For this review, take the finished solid that the model builds, in its own axes (mm). A direction names the side the tool comes from. Round coordinates to 2 decimals unless told otherwise and drop trailing zeros. Loops run counter-clockwise (first coordinate to the right, second up) from the corner with the lowest first, then second, coordinate; pieces in that order, holes last.
1. Tool access review of faces 1 (the flat face through (-9, 4.5, 0)), 2 (the flat face through (-2, 26.7, 0)), 3 (the flat face through (15, 17, 0.65)): name each direction out of +Z, -Z, +X, -X, +Y, -Y from which nothing blocks a thin tool from reaching the whole face with its end or side.
2. Clearance check with flat-ended pins moving along their axes: pin 1 Ø2 at (y, z) = (23.5, 3) entering from -X; pin 2 Ø4.5 at (y, z) = (20, 2.5) entering from -X; pin 3 Ø6 at (x, z) = (4.5, 1) entering from +Y; pin 4 Ø1.4 at (x, z) = (-14.5, -2) entering from +Y. State where each tip first meets the part, or that it passes through.
3. To check wall thickness, follow line 1 along Y through (x, z) = (-10, 0.25); line 2 along Z through (x, y) = (-13.65, 17.2); line 3 along X through (y, z) = (17.15, 0). State the ranges of each line that lie inside material, in increasing order.
4. Consider section C-C on x = 0.95. State the section outline as (y, z) points, then the cut area to 3 significant figures.
5. Consider section D-D on y = 13.75. State the section outline as (x, z) points.
6. Consider section A-A on x = 13.65. State the section outline as (y, z) points, then the cut area to 3 significant figures.
7. Consider section B-B on z = -3.25. State the section outline as (x, y) points, then the cut area to 3 significant figures.
from build123d import *

# Parameters (mm, degrees)
SKETCH1_W           = 22.5
SKETCH1_H           = 11.8
BOSS_EXTRUDE1_DEPTH = 22.7
BOSS_EXTRUDE2_START = 15.9
SKETCH2_W           = 31.9
SKETCH2_H           = 11.8
BOSS_EXTRUDE2_DEPTH = 2.5
SKETCH3_R           = 1
CUT_EXTRUDE1_DEPTH  = 26.055388642
SKETCH4_R           = 5.9
SKETCH4_R_2         = 2.3
SKETCH4_R_3         = 2.5
BOSS_EXTRUDE3_DEPTH = 4
SKETCH4_3_R         = 2.3
BOSS_EXTRUDE4_DEPTH = 7.2
SKETCH5_W           = 3.6
SKETCH5_H           = 1.2
CUT_EXTRUDE2_DEPTH  = 4


with BuildPart() as part:
    # Sketch1 → Boss-Extrude1 (new body)
    with BuildSketch(Plane(origin=(0, 0, 0), x_dir=(1, 0, 0), z_dir=(0, 1, 0))):
        Rectangle(SKETCH1_W, SKETCH1_H)
    extrude(amount=BOSS_EXTRUDE1_DEPTH)

    # Sketch2 → Boss-Extrude2 (add)
    with BuildSketch(Plane(origin=(0, 0, 0), x_dir=(1, 0, 0), z_dir=(0, 1, 0)).offset(BOSS_EXTRUDE2_START)):
        Rectangle(SKETCH2_W, SKETCH2_H)
    extrude(amount=BOSS_EXTRUDE2_DEPTH)

    # Sketch3 → Cut-Extrude1 (cut, through all)
    with BuildSketch(Plane(origin=(0, 18.4, 0), x_dir=(1, 0, 0), z_dir=(0, 1, 0))):
        with BuildLine():
            Line((-14.409934208, 0.65), (-15.95, 0.65))
            Line((-15.95, 0.65), (-15.95, -0.65))
            Line((-15.95, -0.65), (-14.409934208, -0.65))
            ThreePointArc((-14.409934208, -0.65), (-14.65, 0), (-14.409934208, 0.65))
        make_face()
        with Locations((-13.65, 0)):
            Circle(SKETCH3_R)
        with Locations((13.65, 0)):
            Circle(SKETCH3_R)
        with BuildLine():
            Line((14.409934208, -0.65), (15.95, -0.65))
            Line((15.95, -0.65), (15.95, 0.65))
            Line((15.95, 0.65), (14.409934208, 0.65))
            ThreePointArc((14.409934208, 0.65), (14.588065618, 0.34645764), (14.65, 0))
            ThreePointArc((14.65, 0), (14.588065618, -0.34645764), (14.409934208, -0.65))
        make_face()
    extrude(amount=-CUT_EXTRUDE1_DEPTH, mode=Mode.SUBTRACT)

    # Sketch4 → Boss-Extrude3 (add)
    # profile 1 of 2: a face of its own
    with BuildSketch(Plane(origin=(0, 22.7, 0), x_dir=(1, 0, 0), z_dir=(0, 1, 0))):
        with Locations((-5.35, 0)):
            Circle(SKETCH4_R)
        with Locations(Location((-5.35, 0, 0), (0, 0, 270))):
            Circle(SKETCH4_R_2, mode=Mode.SUBTRACT)
    # profile 2 of 2: a face of its own
    with BuildSketch(Plane(origin=(0, 22.7, 0), x_dir=(1, 0, 0), z_dir=(0, 1, 0))):
        with Locations((0.95, 0)):
            Circle(SKETCH4_R_3)
    extrude(amount=BOSS_EXTRUDE3_DEPTH)

    # Sketch4_3 → Boss-Extrude4 (add)
    with BuildSketch(Plane(origin=(0, 22.7, 0), x_dir=(1, 0, 0), z_dir=(0, 1, 0))):
        with Locations(Location((-5.35, 0, 0), (0, 0, 270))):
            Circle(SKETCH4_3_R)
    extrude(amount=BOSS_EXTRUDE4_DEPTH)

    # Sketch5 → Cut-Extrude2 (cut)
    with BuildSketch(Plane.ZY.offset(11.25)):
        with Locations((0, 5.1)):
            Rectangle(SKETCH5_W, SKETCH5_H)
    extrude(amount=-CUT_EXTRUDE2_DEPTH, mode=Mode.SUBTRACT)


solid = part.part
Resolved:
1. face 1: -X
1. face 2: +Y
1. face 3: +X, +Y, -Y
2. pin 1: stops at x = -11.25
2. pin 2: stops at x = -15.95
2. pin 3: stops at y = 26.7
2. pin 4: stops at y = 18.4
3. line 1: y = 0 to 4.5, 5.7 to 26.7
3. line 2: z = -5.9 to -1, 1 to 5.9
3. line 3: x = -12.65 to 12.65
4. outline: (0, -5.9) - (22.7, -5.9) - (22.7, -2.5) - (26.7, -2.5) - (26.7, 2.5) - (22.7, 2.5) - (22.7, 5.9) - (0, 5.9) - close
4. area: 288 mm2
5. outline: (-11.25, -5.9) - (11.25, -5.9) - (11.25, 5.9) - (-11.25, 5.9) - close
6. outline: (15.9, -5.9) - (18.4, -5.9) - (18.4, -1) - (15.9, -1) - close; (15.9, 1) - (18.4, 1) - (18.4, 5.9) - (15.9, 5.9) - close
6. area: 24.5 mm2
7. outline: (-15.95, 15.9) - (-11.25, 15.9) - (-11.25, 0) - (11.25, 0) - (11.25, 15.9) - (15.95, 15.9) - (15.95, 18.4) - (11.25, 18.4) - (11.25, 22.7) - (-0.43, 22.7) - (-0.43, 26.7) - (-10.27, 26.7) - (-10.27, 22.7) - (-11.25, 22.7) - (-11.25, 18.4) - (-15.95, 18.4) - close
7. area: 574 mm2
